The figure shows three views and two pictorial views of one solid part (mm, origin at its lowest corner). Answer the questions. A direction names the side the tool comes from. Coordinates: 2 decimals unless noted, no trailing zeros. Loops run counter-clockwise (first coordinate to the right, second up) from the corner with the lowest first, then second, coordinate; pieces in that order, holes last.
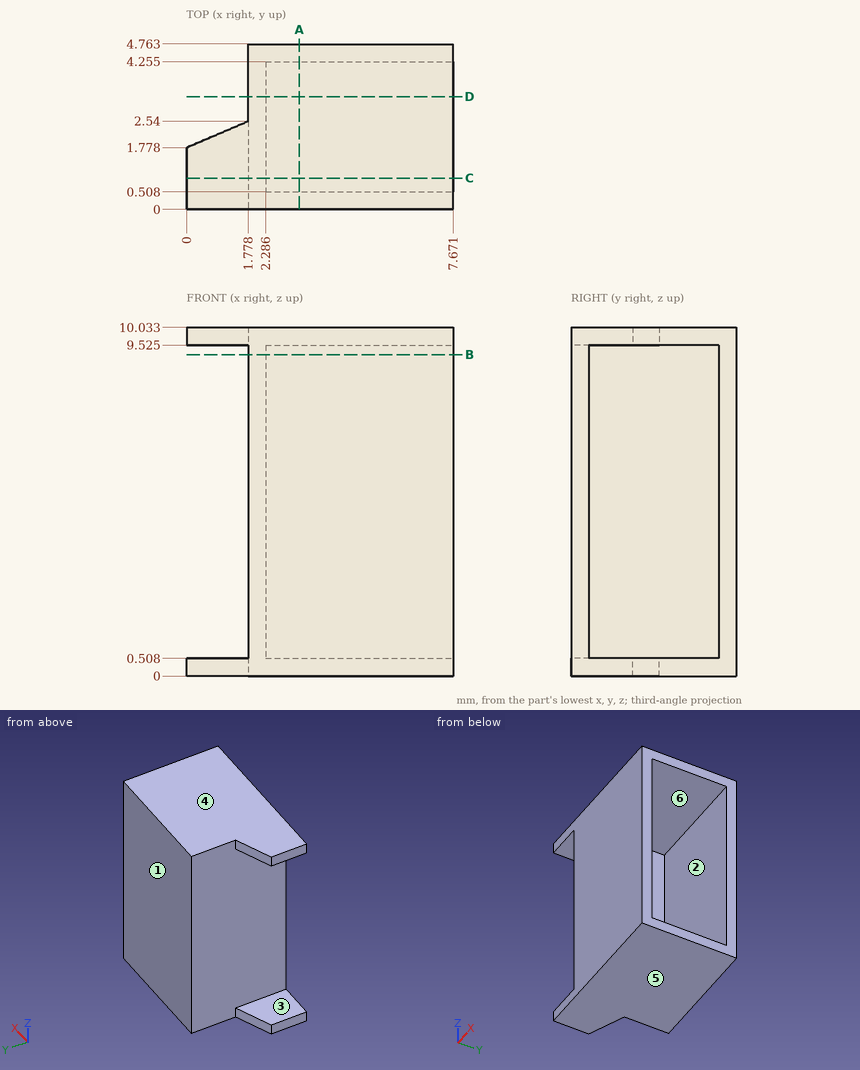
Q1. A cutting plane is placed at D-D (y = 3.25). Give the vertices of the cut face in (x, z) (1 decimal).
Findings below:
outline: (1.8, 0) - (7.7, 0) - (7.7, 0.5) - (2.3, 0.5) - (2.3, 9.5) - (7.7, 9.5) - (7.7, 10) - (1.8, 10) - close
Q2. Straight lines are drawn through the part: probe 1 along Y at (x, z) = (5, 2.5) (1 decimal); probe 2 along Z at (x, y) = (7.25, 0.9) (1 decimal); probe 3 along X at (y, z) = (3.9, 3.25) (1 decimal). For each, find the intervals that lie inside material, in ascending order.
Findings below:
probe 1: y = 0 to 0.5, 4.3 to 4.8
probe 2: z = 0 to 0.5, 9.5 to 10
probe 3: x = 1.8 to 2.3
Q3. Which of the six approach directions +Z, -Z, +X, -X, +Y, -Y give full straight-line access (tool end or side, diameter ignored) to the marked faces 1, 2 and 3?
Findings below:
face 1: +Z, -Z, +X, -X, +Y
face 2: +X
face 3: -X, +Y, -Y
Q4. A cutting plane is placed at C-C (y = 0.9). Give the vertices of the cut face in (x, z) (1 decimal).
Findings below:
outline: (0, 0) - (7.7, 0) - (7.7, 0.5) - (2.3, 0.5) - (2.3, 9.5) - (7.7, 9.5) - (7.7, 10) - (0, 10) - (0, 9.5) - (1.8, 9.5) - (1.8, 0.5) - (0, 0.5) - close
Q5. Determine the mould class of the marked faces 4, 5 and 6 for opening direction Z: +Z half, -Z half, draft (parallel to the pull), parting line (faces both ways), or undercut.
Findings below:
face 4: +Z half
face 5: -Z half
face 6: undercut
Q6. Flat-ended cylindrical pins translate along their axes: pin 1 Ø1 at (y, z) = (1, 6.5) entering from -X; pin 2 Ø2 at (x, y) = (1, 1) entering from -Z. Find the tip coordinate at first contact, or state that the pin passes through.
Findings below:
pin 1: stops at x = 1.78
pin 2: stops at z = 0
Q7. A cutting plane is placed at B-B (z = 9.25). Give the vertices of the cut face in (x, y) (1 decimal).
Findings below:
outline: (1.8, 0) - (7.7, 0) - (7.7, 0.5) - (2.3, 0.5) - (2.3, 4.3) - (7.7, 4.3) - (7.7, 4.8) - (1.8, 4.8) - close
Q8. A cutting plane is placed at A-A (x = 3.25). Give the vertices of the cut face in (y, z) (1 decimal).
Findings below:
outline: (0, 0) - (4.8, 0) - (4.8, 10) - (0, 10) - close; hole (0.5, 0.5) - (4.3, 0.5) - (4.3, 9.5) - (0.5, 9.5) - close
